Check sheet for the modelled part. Datum: model origin and axes. Units: mm. A direction names the side the tool comes from. Coordinates: 2 decimals unless noted, no trailing zeros. Loops run counter-clockwise (first coordinate to the right, second up) from the corner with the lowest first, then second, coordinate; pieces in that order, holes last.
```python
from build123d import *

# Parameters (mm, degrees)
SKETCH1_R           = 2
SKETCH1_R_2         = 0.5
BOSS_EXTRUDE1_DEPTH = 9.5
SKETCH1_3_R         = 2
SKETCH1_3_R_2       = 0.5
CUT_EXTRUDE1_DEPTH  = 6.5
BOSS_EXTRUDE2_DEPTH = 3
CUT_EXTRUDE2_START  = 20
SKETCH3_R           = 2.25
CUT_EXTRUDE2_DEPTH  = 6
SKETCH5_R           = 1.6
CUT_EXTRUDE3_DEPTH  = 10


with BuildPart() as part:
    # Sketch1 → Boss-Extrude1 (new body)
    with BuildSketch(Plane(origin=(0, 0, 0), x_dir=(0, 0, -1), z_dir=(1, 0, 0))):
        with BuildLine():
            Line((2.814717913, -14.792070209), (10.42585747, -7.09701164))
            ThreePointArc((10.42585747, -7.09701164), (9.72468907, -5.811561885), (8.865865393, -4.625627615))
            ThreePointArc((8.865865393, -4.625627615), (9.731180291, 2.303069722), (5.85199823, 8.108891213))
            ThreePointArc((5.85199823, 8.108891213), (0, 18.95), (-5.85199823, 8.108891213))
            ThreePointArc((-5.85199823, 8.108891213), (-9.731180291, 2.303069722), (-8.865865393, -4.625627615))
            ThreePointArc((-8.865865393, -4.625627615), (-9.72468907, -5.811561885), (-10.42585747, -7.09701164))
            Line((-10.42585747, -7.09701164), (-2.814717913, -14.792070209))
            ThreePointArc((-2.814717913, -14.792070209), (0, -15.95), (2.814717913, -14.792070209))
        make_face()
        with Locations((0, -11.95)):
            Circle(SKETCH1_R, mode=Mode.SUBTRACT)
        Circle(SKETCH1_R, mode=Mode.SUBTRACT)
        with Locations((0, 11.95)):
            Circle(SKETCH1_R_2, mode=Mode.SUBTRACT)
        with BuildLine():
            Line((10.42585747, -7.09701164), (12.5, -5))
            Line((12.5, -5), (12.5, 20))
            Line((12.5, 20), (-12.5, 20))
            Line((-12.5, 20), (-12.5, -5))
            Line((-12.5, -5), (-10.42585747, -7.09701164))
            ThreePointArc((-10.42585747, -7.09701164), (-9.72468907, -5.811561885), (-8.865865393, -4.625627615))
            ThreePointArc((-8.865865393, -4.625627615), (-9.731180291, 2.303069722), (-5.85199823, 8.108891213))
            ThreePointArc((-5.85199823, 8.108891213), (0, 18.95), (5.85199823, 8.108891213))
            ThreePointArc((5.85199823, 8.108891213), (9.731180291, 2.303069722), (8.865865393, -4.625627615))
            ThreePointArc((8.865865393, -4.625627615), (9.72468907, -5.811561885), (10.42585747, -7.09701164))
        make_face()
    extrude(amount=BOSS_EXTRUDE1_DEPTH)

    # Sketch1<3> → Cut-Extrude1 (cut)
    with BuildSketch(Plane(origin=(0, 0, 0), x_dir=(0, 0, -1), z_dir=(1, 0, 0))):
        with BuildLine():
            Line((2.814717913, -14.792070209), (10.42585747, -7.09701164))
            ThreePointArc((10.42585747, -7.09701164), (9.72468907, -5.811561885), (8.865865393, -4.625627615))
            ThreePointArc((8.865865393, -4.625627615), (9.731180291, 2.303069722), (5.85199823, 8.108891213))
            ThreePointArc((5.85199823, 8.108891213), (0, 18.95), (-5.85199823, 8.108891213))
            ThreePointArc((-5.85199823, 8.108891213), (-9.731180291, 2.303069722), (-8.865865393, -4.625627615))
            ThreePointArc((-8.865865393, -4.625627615), (-9.72468907, -5.811561885), (-10.42585747, -7.09701164))
            Line((-10.42585747, -7.09701164), (-2.814717913, -14.792070209))
            ThreePointArc((-2.814717913, -14.792070209), (0, -15.95), (2.814717913, -14.792070209))
        make_face()
        with Locations((0, -11.95)):
            Circle(SKETCH1_3_R, mode=Mode.SUBTRACT)
        Circle(SKETCH1_3_R, mode=Mode.SUBTRACT)
        with Locations((0, 11.95)):
            Circle(SKETCH1_3_R_2, mode=Mode.SUBTRACT)
    extrude(amount=CUT_EXTRUDE1_DEPTH, mode=Mode.SUBTRACT)

    # Sketch4 → Boss-Extrude2 (add)
    with BuildSketch(Plane(origin=(0, 0, 0), x_dir=(0, 0, -1), z_dir=(1, 0, 0))):
        with BuildLine():
            Line((4.898979486, 16.95), (-4.898979486, 16.95))
            ThreePointArc((-4.898979486, 16.95), (0, 18.95), (4.898979486, 16.95))
        make_face()
    extrude(amount=BOSS_EXTRUDE2_DEPTH)

    # Sketch3 → Cut-Extrude2 (cut)
    with BuildSketch(Plane(origin=(0, 0, 0), x_dir=(1, 0, 0), z_dir=(0, 1, 0)).offset(CUT_EXTRUDE2_START)):
        Circle(SKETCH3_R)
    extrude(amount=-CUT_EXTRUDE2_DEPTH, mode=Mode.SUBTRACT)

    # Sketch5 → Cut-Extrude3 (cut)
    with BuildSketch(Plane(origin=(0, 0, 0), x_dir=(0, 0, -1), z_dir=(1, 0, 0))):
        with Locations((9.5, 9)):
            Circle(SKETCH5_R)
        with Locations((-9.5, 9)):
            Circle(SKETCH5_R)
        with Locations((-9.5, 17)):
            Circle(SKETCH5_R)
        with Locations((9.5, 17)):
            Circle(SKETCH5_R)
    extrude(amount=CUT_EXTRUDE3_DEPTH, mode=Mode.SUBTRACT)


solid = part.part
```
1) Depth check by flat-ended pin: pin 1 (3 mm diameter, centred on y = -11.95, z = 0, fed in from +X); pin 2 (1.5 mm diameter, centred on x = 1, z = -2.5, fed in from -Y); pin 3 (4 mm diameter, centred on x = 1.5, y = -8, fed in from -Z); pin 4 (10.5 mm diameter, centred on y = 9, z = -0.5, fed in from -X). Enter the tip coordinate at first touch or a pass-through.
Answer sheet:
pin 1: passes through
pin 2: stops at y = 16.95
pin 3: stops at z = -11.51
pin 4: stops at x = 6.5
2) Scan lines: line 1 (Z direction, x = 7, y = 9); line 2 (Y direction, x = 7.2, z = 0); line 3 (Z direction, x = 4.5, y = 17). Record each from-to range of solid material in increasing order.
Answer sheet:
line 1: z = -12.5 to -11.1, -7.9 to 7.9, 11.1 to 12.5
line 2: y = -15.95 to -13.95, -9.95 to -2, 2 to 11.45, 12.45 to 20
line 3: z = -12.5 to -11.1, -7.9 to -4.85, 4.85 to 7.9, 11.1 to 12.5
3) Section check A-A on y = 11.95. Enter the section's corners in (x, z).
Answer sheet:
outline: (0, -12.5) - (9.5, -12.5) - (9.5, -0.5) - (6.5, -0.5) - (6.5, -7) - (0, -7) - close; (0, 7) - (6.5, 7) - (6.5, 0.5) - (9.5, 0.5) - (9.5, 12.5) - (0, 12.5) - close
4) Section check D-D on x = 8.25. Enter the section's corners in (y, z), plus the area to 3 significant figures.
Answer sheet:
outline: (-14.79, -2.81) - (-5, -12.5) - (20, -12.5) - (20, 12.5) - (-5, 12.5) - (-14.79, 2.81) arc R4 ccw to start; hole circle Ø4 at (-11.95, 0); hole circle Ø4 at (0, 0); hole circle Ø3.2 at (9, -9.5); hole circle Ø3.2 at (9, 9.5); hole circle Ø1 at (11.95, 0); hole circle Ø3.2 at (17, -9.5); hole circle Ø3.2 at (17, 9.5)
area: 721 mm2
5) Set-up check for faces 1 (the cylindrical face through (3.2, -5.79, 9.71)), 2 (the cylindrical face through (3.204, 2.4, 9.708)), 3 (the cylindrical face through (3.204, 18.947, -0.211)): record each of +Z, -Z, +X, -X, +Y, -Y from which the full face is reachable in a straight line by a thin tool's end or side.
Answer sheet:
face 1: -X, -Y
face 2: -X
face 3: none
6) Section check C-C on x = 4. Enter the section's corners in (y, z), plus the area to 3 significant figures.
Answer sheet:
outline: (-7.1, -10.43) - (-5, -12.5) - (20, -12.5) - (20, 12.5) - (-5, 12.5) - (-7.1, 10.43) arc R11.5 cw to (-4.63, 8.87) arc R10 cw to (8.11, 5.85) arc R7 cw (long way) to (8.11, -5.85) arc R10 cw to (-4.63, -8.87) arc R11.5 cw to start; hole circle Ø3.2 at (9, -9.5); hole circle Ø3.2 at (9, 9.5); hole circle Ø3.2 at (17, -9.5); hole circle Ø3.2 at (17, 9.5)
area: 234 mm2
7) Mould release check, pull along X, two halves, no side actions. Record for faces 4 (the flat face through (0, 10, -7)), 5 (the flat face through (9.5, 6, 0)), 6 (the flat face through (3, 18, 0)): +X half, -X half, draft (parallel to the pull), parting line (faces both ways), or undercut.
Answer sheet:
face 4: -X half
face 5: +X half
face 6: undercut
8) Section check B-B on z = 0. Enter the section's corners in (x, y).
Answer sheet:
outline: (2.25, 16.95) - (3, 16.95) - (3, 18.95) - (6.5, 18.95) - (6.5, 12.45) - (9.5, 12.45) - (9.5, 20) - (2.25, 20) - close; (6.5, -15.95) - (9.5, -15.95) - (9.5, -13.95) - (6.5, -13.95) - close; (6.5, -9.95) - (9.5, -9.95) - (9.5, -2) - (6.5, -2) - close; (6.5, 2) - (9.5, 2) - (9.5, 11.45) - (6.5, 11.45) - close
